Check sheet for the drawn part. Datum: minimum x, y, z corner. Units: mm. A direction names the side the tool comes from. Give positions to 0.01 mm unless a question says otherwise; leave off trailing zeros. Write each loop counter-clockwise with the first axis right and the second up, starting at its lowest first coordinate (ties: lowest second). Pieces come first, ordered by that corner, then holes.
(1) Cross-section at C-C (y = 72.5). Record the boundary of the cut face in (x, z), and give its area (3 significant figures).
(2) Cross-section at D-D (y = 64). Record the boundary of the cut face in (x, z).
(3) Tool access check on the marked faces 4, 5, 6 and 7. Record the directions out of +Z, -Z, +X, -X, +Y, -Y that give a thin tool (end or side, any length) a straight path to the whole face; none if there is none.
(4) Depth check by flat-ended pin: P1, Ø10, axis at y = 13.5, z = 139.5, coming from the +X side; P2, Ø9.5, axis at x = 32, z = 114.5, coming from the +Y side; P3, Ø21.5, axis at y = 40, z = 69, coming from the +X side; P4, Ø24, axis at x = 26.5, y = 36.5, coming from the +Z side. Enter the tip coordinate at first touch or a pass-through.
(5) Thickness scan on line 1 along Y through (x, z) = (46, 30); line 2 along X through (y, z) = (8, 26); line 3 along Y through (x, z) = (51, 83.5). Record the ranges inside material, lowest first.
(6) Cross-section at B-B (z = 34). Record the boundary of the cut face in (x, y).
(7) Mould release check, pull along Z, two halves, no side actions. Record for the marked faces 1, 2 and 3: +Z half, -Z half, draft (parallel to the pull), parting line (faces both ways), or undercut.
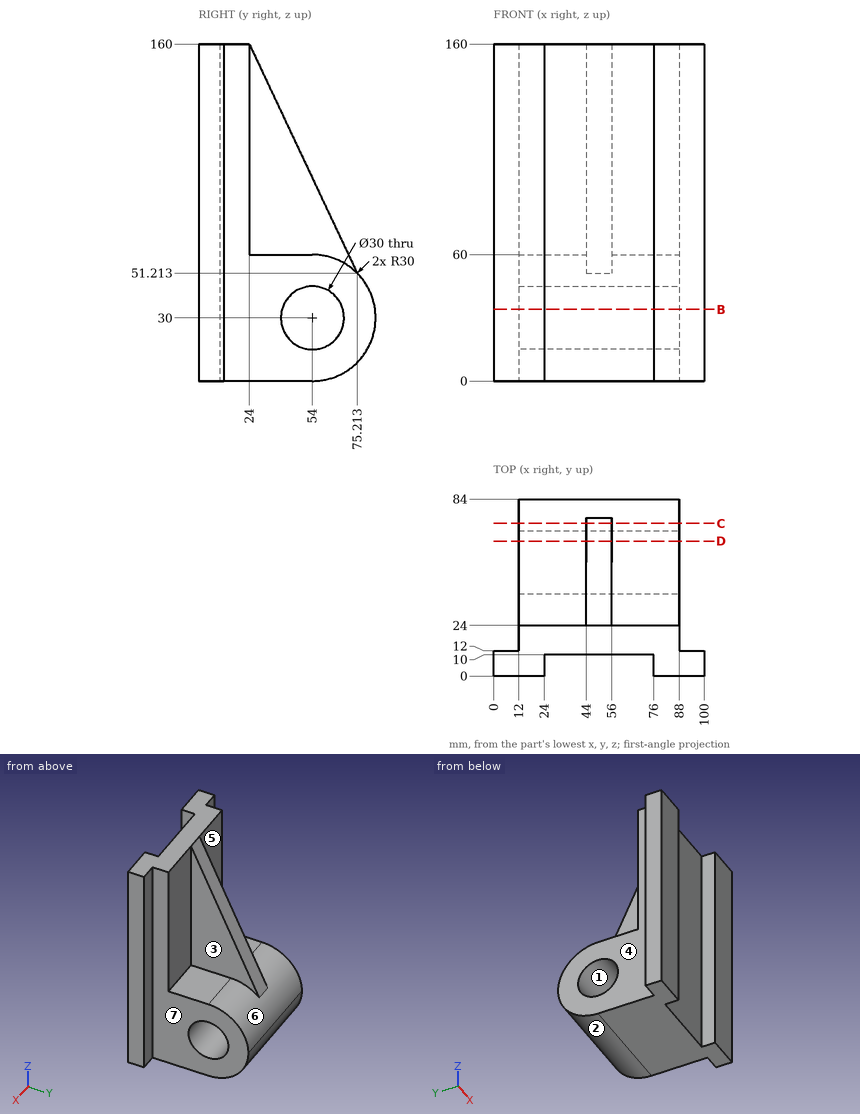
Reply:
1. outline: (12, 6.38) - (88, 6.38) - (88, 53.62) - (56, 53.62) - (56, 56.98) - (44, 56.98) - (44, 53.62) - (12, 53.62) - close
1. area: 3,630 mm2
2. outline: (12, 1.72) - (88, 1.72) - (88, 18.82) - (12, 18.82) - close; (12, 41.18) - (88, 41.18) - (88, 58.28) - (56, 58.28) - (56, 75.03) - (44, 75.03) - (44, 58.28) - (12, 58.28) - close
3. face 4: +Z, -Z, -X, +Y
3. face 5: +Z, -X, +Y
3. face 6: +Z, +Y
3. face 7: +Z, -Z, +X, +Y
4. P1: stops at x = 100
4. P2: stops at y = 24
4. P3: stops at x = 88
4. P4: stops at z = 60
5. line 1: y = 10 to 39, 69 to 84
5. line 2: x = 0 to 24, 76 to 100
5. line 3: y = 10 to 60.01
6. outline: (0, 0) - (24, 0) - (24, 10) - (76, 10) - (76, 0) - (100, 0) - (100, 12) - (88, 12) - (88, 39.54) - (12, 39.54) - (12, 12) - (0, 12) - close; (12, 68.46) - (88, 68.46) - (88, 83.73) - (12, 83.73) - close
7. face 1: undercut
7. face 2: -Z half
7. face 3: draft
